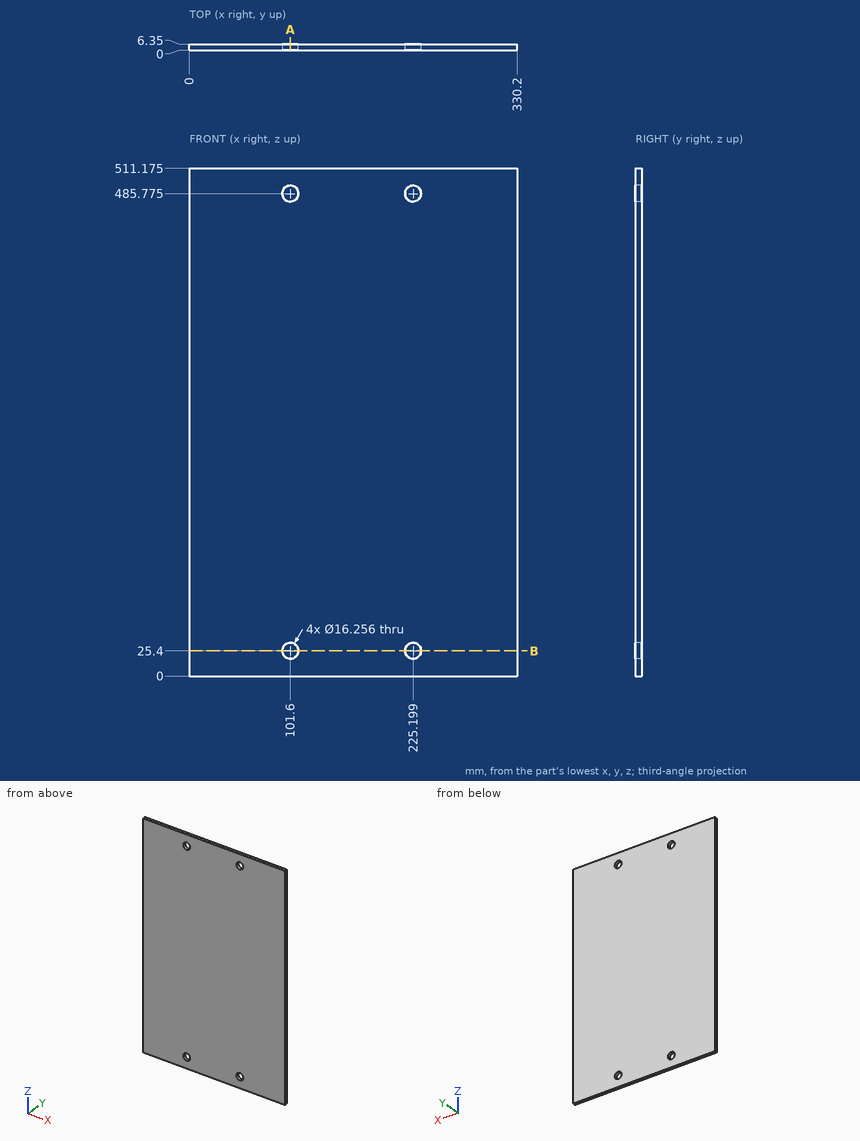
Part print with two shaded views. Sizes in mm from the minimum x, y, z corner. Give positions to 0.01 mm unless a question says otherwise; leave off trailing zeros. Order: outer loops, then holes, each group sorted by start corner. A loop starts at its lowest first (then second) coordinate and runs counter-clockwise, first axis right, second up.
(1) Saw through at A-A, the plane x = 101.6. Give the cut face in (y, z) (3 decimals), then the cut area to 3 significant figures.
(2) Drill centre lines: L1, parallel to Z at x = 101.6, y = 3 (3 decimals); L2, parallel to Z at x = 97, y = 5.5 (1 decimal). Where is each one in solid material? Low to high.
(3) Flat gauge pin, fed straight in: pin 1 (10 mm diameter, centred on x = 101.6, z = 25.4, fed in from +Y). Where does the tip first touch, or does it go through?
(4) Saw through at B-B, the plane z = 25.4. Give the cut face in (x, y), then the cut area to 3 significant figures.
Results found:
1. outline: (0, 0) - (6.35, 0) - (6.35, 17.272) - (0, 17.272) - close; (0, 33.528) - (6.35, 33.528) - (6.35, 477.647) - (0, 477.647) - close; (0, 493.903) - (6.35, 493.903) - (6.35, 511.175) - (0, 511.175) - close
1. area: 3,040 mm2
2. L1: z = 0 to 17.272, 33.528 to 477.647, 493.903 to 511.175
2. L2: z = 0 to 18.7, 32.1 to 479.1, 492.5 to 511.2
3. pin 1: passes through
4. outline: (0, 0) - (93.47, 0) - (93.47, 6.35) - (0, 6.35) - close; (109.73, 0) - (217.07, 0) - (217.07, 6.35) - (109.73, 6.35) - close; (233.33, 0) - (330.2, 0) - (330.2, 6.35) - (233.33, 6.35) - close
4. area: 1,890 mm2
